Source: three-view drawing plus pictorial views. Frame: mm from the lowest corner of the part. A direction names the side the tool comes from. Coordinates: 2 decimals unless noted, no trailing zeros. Loops run counter-clockwise (first coordinate to the right, second up) from the corner with the lowest first, then second, coordinate; pieces in that order, holes last. Notation, with made-up numbers: M -0.75,-37.75 L 40.25,-37.75 A15 cw 40.25,-19.75 Z; hole C -14.5,70.5 d10. An arc over 180 degrees is marked long. Use a Markdown table: item, result. Add a question column.
1. Set-up query: the marked faces 1 and 2. Return all of +Z, -Z, +X, -X, +Y, -Y with unobstructed straight access to the full face (end or side cutting, diameter ignored); none if empty.
2. Pin query (flat end, axial travel): pin 1 (1.5 mm diameter, centred on x = 71.5, z = 21, fed in from -Y). Return the tip coordinate at first contact, or that it passes through.
3. Draft query along Z for the marked faces 3, 4 and 5. Return one class per face: +Z half, -Z half, draft (parallel to the pull), parting line (faces both ways), or undercut.
4. Section D-D on x = 9. Output: boundary loops of the cut face in (y, z) (1 decimal).
5. Section B-B on y = 66. Output: boundary loops of the cut face in (x, z) (1 decimal), then the cut area to 3 significant figures.
6. Section A-A on x = 24.5. Output: boundary loops of the cut face in (y, z).
7. Line query: L1, parallel to Z at x = 9.5, y = 77.5; L2, parallel to Y at x = 37, z = 20 (1 decimal); L3, parallel to Y at x = 59.5, z = 41 (1 decimal). Output: solid intervals per line, ascending. Write a range as [from, to].
8. Section C-C on z = 29. Output: boundary loops of the cut face in (x, y) (1 decimal).
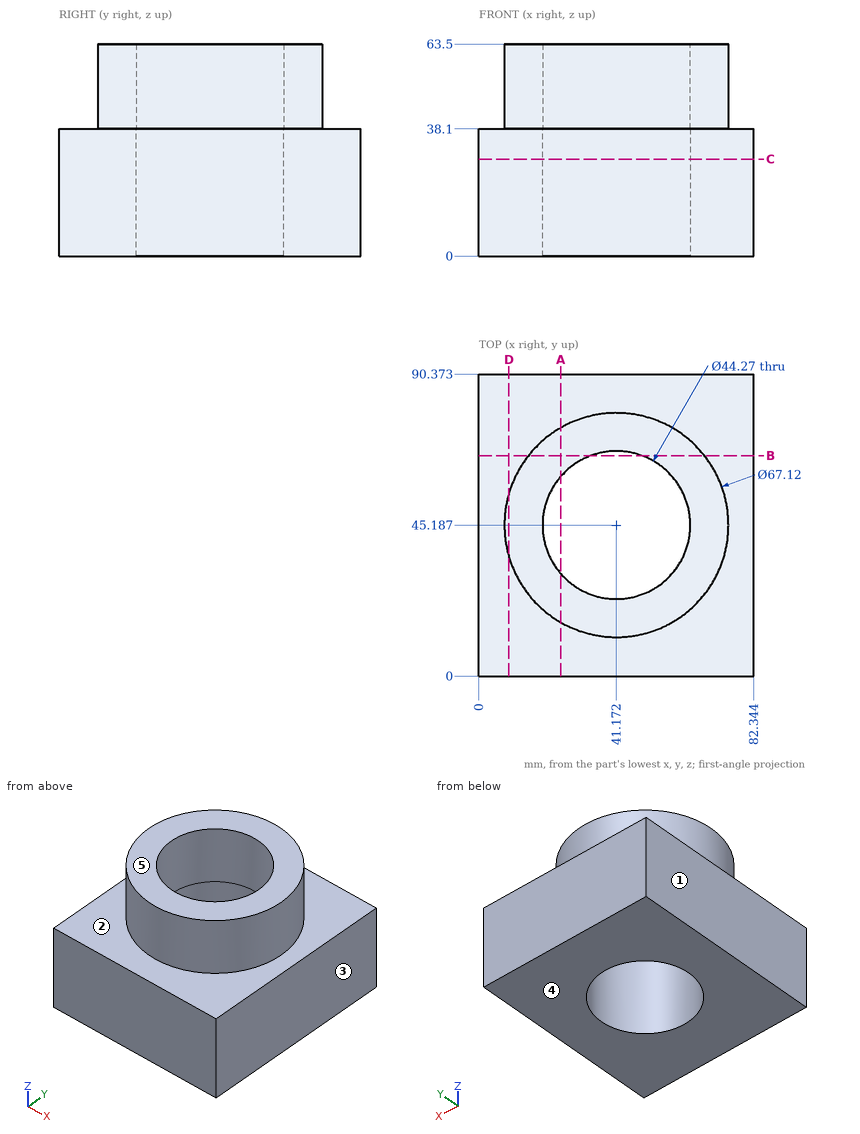
Answers below:
| question | item | result |
|---|---|---|
| 1 | face 1 | +Z, -Z, -X, +Y, -Y |
| 1 | face 2 | +Z |
| 2 | pin 1 | stops at y = 0 |
| 3 | face 3 | draft |
| 3 | face 4 | -Z half |
| 3 | face 5 | +Z half |
| 4 | outline | M 0,0 L 90.4,0 L 90.4,38.1 L 54.7,38.1 L 54.7,63.5 L 35.6,63.5 L 35.6,38.1 L 0,38.1 Z |
| 5 | outline | M 0,0 L 33.6,0 L 33.6,63.5 L 14.8,63.5 L 14.8,38.1 L 0,38.1 Z; M 48.7,0 L 82.3,0 L 82.3,38.1 L 67.5,38.1 L 67.5,63.5 L 48.7,63.5 Z |
| 5 | area | 3,520 mm² |
| 6 | outline | M 0,0 L 30.63,0 L 30.63,63.5 L 16.06,63.5 L 16.06,38.1 L 0,38.1 Z; M 59.75,0 L 90.37,0 L 90.37,38.1 L 74.31,38.1 L 74.31,63.5 L 59.75,63.5 Z |
| 7 | L1 | z = [0, 38.1] |
| 7 | L2 | y = [0, 23.4], [66.9, 90.4] |
| 7 | L3 | y = [17.1, 32.8], [57.6, 73.3] |
| 8 | outline | M 0,0 L 82.3,0 L 82.3,90.4 L 0,90.4 Z; hole C 41.2,45.2 d44.3 |
